Geometry check sheet. Reference: the model listing, model coordinates, mm. Face numbers are marked on the shaded views. A direction names the side the tool comes from. Coordinates: 2 decimals unless noted, no trailing zeros. Order: outer loops, then holes, each group sorted by start corner. A loop starts at its lowest first (then second) coordinate and runs counter-clockwise, first axis right, second up.
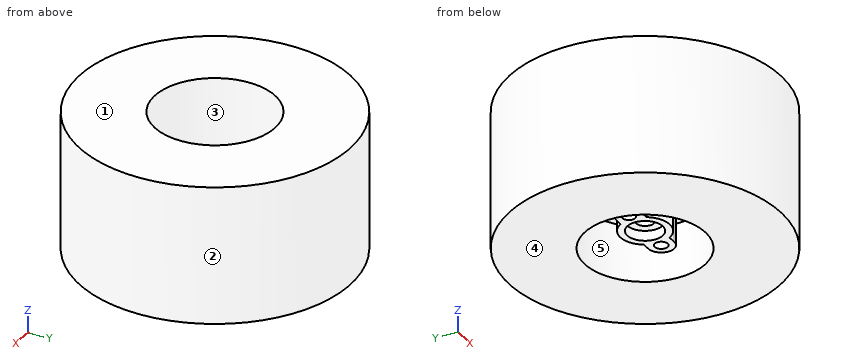
```python
from build123d import *

# Parameters (mm, degrees)
SKETCH_R        = 36.576
PAD_DEPTH       = 37.1475
SKETCH001_R     = 16.256
POCKET_DEPTH    = 19.9771
SKETCH002_R     = 16.256
POCKET001_DEPTH = 14.8463
PAD001_DEPTH    = 10.1219
SKETCH004_R     = 1.74625
POCKET002_DEPTH = 32.4241
SKETCH005_R     = 4.7879
POCKET003_DEPTH = 2.6924
SKETCH006_R     = 2.425304
POCKET004_DEPTH = 29.7317
SKETCH007_R     = 4.7879
POCKET005_DEPTH = 3.1242


with BuildPart() as part:
    # Sketch → Pad (new body)
    with BuildSketch(Plane.XY):
        Circle(SKETCH_R)
    extrude(amount=PAD_DEPTH)

    # Sketch001 (on Face3 of Pad) → Pocket (cut)
    with BuildSketch(Plane.XY.offset(37.1475)):
        Circle(SKETCH001_R)
    extrude(amount=-POCKET_DEPTH, mode=Mode.SUBTRACT)

    # Sketch002 (on Face2 of Pocket) → Pocket001 (cut)
    with BuildSketch(Plane(origin=(0, 0, 0), x_dir=(1, 0, 0), z_dir=(0, 0, -1))):
        Circle(SKETCH002_R)
    extrude(amount=-POCKET001_DEPTH, mode=Mode.SUBTRACT)

    # Sketch003 (on Face6 of Pocket001) → Pad001 (new body)
    with BuildSketch(Plane(origin=(0, 0, 14.8463), x_dir=(1, 0, 0), z_dir=(0, 0, -1))):
        with BuildLine():
            ThreePointArc((-5.67159, -3.48615), (0, -6.65734), (5.67159, -3.48615))
            Line((5.67159, -3.48615), (7.95655, -3.48615))
            ThreePointArc((7.95655, -3.48615), (11.4427, 0), (7.95655, 3.48615))
            Line((5.67159, 3.48615), (7.95655, 3.48615))
            ThreePointArc((5.67159, 3.48615), (0, 6.65734), (-5.67159, 3.48615))
            Line((-7.95655, 3.48615), (-5.67159, 3.48615))
            ThreePointArc((-7.95655, 3.48615), (-11.4427, 0), (-7.95655, -3.48615))
            Line((-7.95655, -3.48615), (-5.67159, -3.48615))
        make_face()
    extrude(amount=PAD001_DEPTH)

    # Sketch004 (on Face16 of Pad001) → Pocket002 (cut, through all)
    with BuildSketch(Plane(origin=(0, 0, 4.7244), x_dir=(1, 0, 0), z_dir=(0, 0, -1))):
        with Locations((7.95782, 0)):
            Circle(SKETCH004_R)
        with Locations((-7.95782, 0)):
            Circle(SKETCH004_R)
    extrude(amount=-POCKET002_DEPTH, mode=Mode.SUBTRACT)

    # Sketch005 (on Face18 of Pocket002) → Pocket003 (cut)
    with BuildSketch(Plane(origin=(0, 0, 4.7244), x_dir=(1, 0, 0), z_dir=(0, 0, -1))):
        Circle(SKETCH005_R)
    extrude(amount=-POCKET003_DEPTH, mode=Mode.SUBTRACT)

    # Sketch006 (on Face20 of Pocket003) → Pocket004 (cut, through all)
    with BuildSketch(Plane(origin=(0, 0, 7.4168), x_dir=(1, 0, 0), z_dir=(0, 0, -1))):
        Circle(SKETCH006_R)
    extrude(amount=-POCKET004_DEPTH, mode=Mode.SUBTRACT)

    # Sketch007 (on Face7 of Pocket004) → Pocket005 (cut)
    with BuildSketch(Plane.XY.offset(17.1704)):
        Circle(SKETCH007_R)
    extrude(amount=-POCKET005_DEPTH, mode=Mode.SUBTRACT)


solid = part.part
```
Item 1: Thickness scan on line 1 along Y through (x, z) = (0, 15); line 2 along Y through (x, z) = (0, 23); line 3 along Z through (x, y) = (6, -7.5). Record the ranges inside material, lowest first.
Item 2: Sectioned sample at A-A (z = 12). Record the cut outline in (x, y), and give its area (3 significant figures).
Item 3: Depth check by flat-ended pin: P1, Ø6.5, axis at x = 4.5, y = 3, coming from the -Z side; P2, Ø1.1, axis at x = 7, z = 10.5, coming from the +Y side; P3, Ø2, axis at y = 20.5, z = 11.5, coming from the -X side; P4, Ø3, axis at x = 7.96, y = 0, coming from the +Z side. Enter the tip coordinate at first touch or a pass-through.
Item 4: Tool access check on the marked faces 4 and 5. Record the directions out of +Z, -Z, +X, -X, +Y, -Y that give a thin tool (end or side, any length) a straight path to the whole face; none if there is none.
Item 5: Sectioned sample at D-D (z = 20.5). Record the cut outline in (x, y).
Item 6: Sectioned sample at C-C (y = 0). Give the number of separate pieces and of enclosed holes in the cut face, and give its area (3 significant figures).
Item 7: Sectioned sample at B-B (x = 0). Record the cut outline in (y, z).
Item 8: Release check for a two-part mould opening along X. For the marked faces 1, 2 and 3 record: pulls with the +X half, pulls with the -X half, needs draft (parallel to the pull), parting line crosses it, or undercut.
Geometry check:
1. line 1: y = -36.58 to -4.79, 4.79 to 36.58
1. line 2: y = -36.58 to -16.26, 16.26 to 36.58
1. line 3: z = 14.85 to 17.17
2. outline: circle Ø73.15 at (0, 0); (-7.96, -3.49) - (-5.67, -3.49) arc R6.66 ccw to (5.67, -3.49) - (7.96, -3.49) arc R3.49 ccw to (7.96, 3.49) - (5.67, 3.49) arc R6.66 ccw to (-5.67, 3.49) - (-7.96, 3.49) arc R3.49 ccw to start; hole circle Ø32.51 at (0, 0); hole circle Ø3.49 at (-7.96, 0); hole circle Ø4.85 at (0, 0); hole circle Ø3.49 at (7.96, 0)
2. area: 3,530 mm2
3. P1: stops at z = 4.72
3. P2: stops at y = 36
3. P3: stops at x = -30.94
3. P4: passes through
4. face 4: -Z, +X, -X, +Y, -Y
4. face 5: -Z
5. outline: circle Ø73.15 at (0, 0); hole circle Ø32.51 at (0, 0)
6. separate pieces: 4
6. enclosed holes: 0
6. area: 1,640 mm2
7. outline: (-36.58, 0) - (-16.26, 0) - (-16.26, 14.85) - (-6.66, 14.85) - (-6.66, 4.72) - (-4.79, 4.72) - (-4.79, 7.42) - (-2.43, 7.42) - (-2.43, 14.05) - (-4.79, 14.05) - (-4.79, 17.17) - (-16.26, 17.17) - (-16.26, 37.15) - (-36.58, 37.15) - close; (2.43, 7.42) - (4.79, 7.42) - (4.79, 4.72) - (6.66, 4.72) - (6.66, 14.85) - (16.26, 14.85) - (16.26, 0) - (36.58, 0) - (36.58, 37.15) - (16.26, 37.15) - (16.26, 17.17) - (4.79, 17.17) - (4.79, 14.05) - (2.43, 14.05) - close
8. face 1: needs draft
8. face 2: parting line crosses it
8. face 3: undercut
